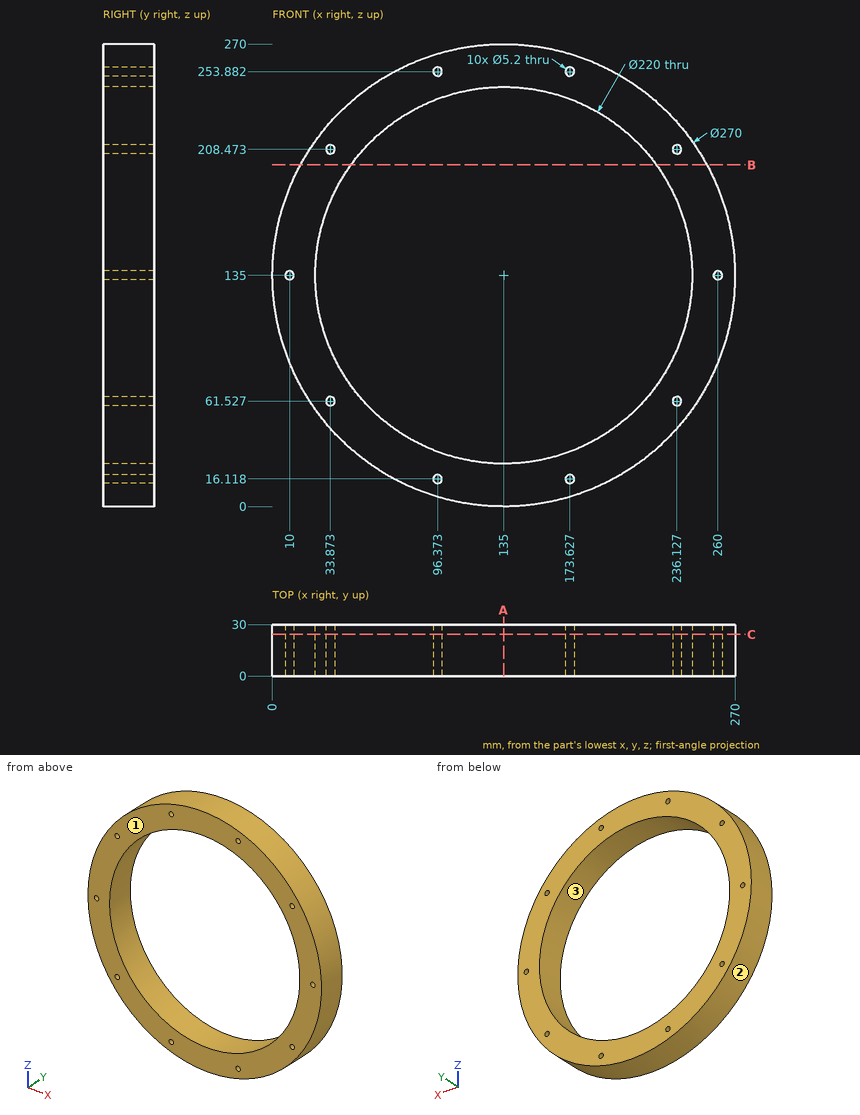
Geometry check sheet. Reference: drawing and pictorial views, mm from the part's lowest x, y, z. Give positions to 0.01 mm unless a question says otherwise; leave off trailing zeros. Loops run counter-clockwise (first coordinate to the right, second up) from the corner with the lowest first, then second, coordinate; pieces in that order, holes last. Notation, with made-up numbers: M 60.25,70 L 84.25,70 A16 cw 84.25,101 Z; hole C 86.5,33 d11. An arc over 180 degrees is marked long. Use a Markdown table: item, result. Add a question column.
Q1. Sectioned sample at C-C, the plane y = 24.25. Give the number of separate pieces and of enclosed holes in the cut face, then the cut area to 3 significant figures.
Q2. Scan lines: line 1 along Z through (x, y) = (135, 22); line 2 along Z through (x, y) = (139.5, 15.25) (3 decimals); line 3 along X through (y, z) = (10.5, 252.5) (1 decimal). Record each from-to range of solid material in increasing order. Write a range as [from, to].
Q3. Go/stop test with flat-tipped pins: pin 1 (4 mm diameter, centred on x = 173.63, z = 253.88, fed in from +Y); pin 2 (5 mm diameter, centred on y = 3.5, z = 58, fed in from +X); pin 3 (8 mm diameter, centred on x = 84.5, y = 20, fed in from -Z); pin 4 (8 mm diameter, centred on x = 161.5, y = 5.5, fed in from +Z). Record where each tip stops, or that it passes through.
Q4. Mould release check, pull along X, two halves, no side actions. Record for the marked faces 1, 2 and 3: pulls with the +X half, pulls with the -X half, needs draft (parallel to the pull), parting line crosses it, or undercut.
Q5. Sectioned sample at B-B, the plane z = 199.5. Record the cut outline in (x, y) (1 decimal), then the cut area to 3 significant figures.
Q6. Sectioned sample at A-A, the plane x = 135. Record the cut outline in (y, z).
Verdict:
| question | item | result |
|---|---|---|
| 1 | separate pieces | 1 |
| 1 | enclosed holes | 11 |
| 1 | area | 19,000 mm^2 |
| 2 | line 1 | [0, 25], [245, 270] |
| 2 | line 2 | [0.075, 25.092], [244.908, 269.925] |
| 2 | line 3 | [68.5, 94.2], [98.6, 171.4], [175.8, 201.5] |
| 3 | pin 1 | through |
| 3 | pin 2 | x = 247.58 |
| 3 | pin 3 | z = 8.26 |
| 3 | pin 4 | z = 268.11 |
| 4 | face 1 | needs draft |
| 4 | face 2 | parting line crosses it |
| 4 | face 3 | undercut |
| 5 | outline | M 16.4,0 L 45.9,0 L 45.9,30 L 16.4,30 Z; M 224.1,0 L 253.6,0 L 253.6,30 L 224.1,30 Z |
| 5 | area | 1,770 mm^2 |
| 6 | outline | M 0,0 L 30,0 L 30,25 L 0,25 Z; M 0,245 L 30,245 L 30,270 L 0,270 Z |
